Source: CAD feature listing. Evaluate the final solid. Frame: model axes, mm. Face numbers are marked on the shaded views. A direction names the side the tool comes from. Give positions to 0.01 mm unless a question says otherwise; leave off trailing zeros. Order: outer loops, then holes, each group sorted by start corner. A loop starts at its lowest first (then second) coordinate and runs counter-clockwise, first axis right, second up. Notation, with made-up numbers: M 37.5,-13 L 79.5,-13 A22 ccw 79.5,-1 Z; hole C -12.75,-14.5 d1. An arc over 180 degrees is marked long. Use CSV: the item, a comma, the result in double quotes. Start each with the question number.
1. Reachability of the marked faces 5, 6, 7 and 8 from +Z, -Z, +X, -X, +Y, -Y: full face, straight path, thin tool, end or side. Return the list, or none.
2. Section query D-D, the plane z = 5. Return the cut outline in (x, y), plus the area to 3 significant figures.
3. Pin query (flat end, axial travel): P1, Ø12, axis at x = -2.5, y = 20.5, coming from the -Z side; P2, Ø1.5, axis at x = -3.5, z = 15.5, coming from the +Y side; P3, Ø6, axis at y = 12.5, z = 8, coming from the +X side; P4, Ø6.5, axis at y = 9.25, z = 10, coming from the +X side. Return the tip coordinate at first contact, or that it passes through.
4. Section query B-B, the plane y = 42. Return the cut outline in (x, z).
5. Mould query, pull axis Y, two halves, no side actions, for the marked faces 1, 2, 3 and 4. Classes: released by +Y, released by -Y, zero draft, split by the parting line, or undercut.
6. Section query A-A, the plane y = 37. Return the cut outline in (x, z), plus the area to 3 significant figures.
7. Line query: line 1 along X through (y, z) = (43, 14.5); line 2 along Y through (x, z) = (11.5, 16); line 3 along Y through (x, z) = (-15, 16.5). Output: solid intervals per line, ascending. Write a range as [from, to].
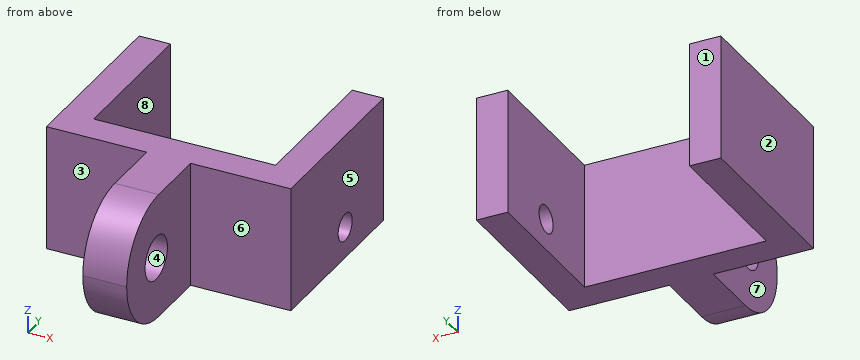
from build123d import *

# Parameters (mm, degrees)
F1_DEPTH = 20
F2_R     = 9.99999
F4_D     = 7
F5_D     = 4.4
F5_DEPTH = 10
F5_TIP   = 1.3218933619


# Not quite as in the source:
# - a fillet or chamfer is up to 0.001 mm smaller than in the source, because OpenCascade refuses the exact size


with BuildPart() as f1:
    # F0 (on Top) → F1 (new body)
    with BuildSketch(Plane.XY):
        Polygon((-18, 49), (-23, 49), (-23, 20), (-7, 20), (-7, 0), (0, 0), (0, 20), (16, 20), (16, 49), (11, 49), (11, 25), (-18, 25), align=None)
    extrude(amount=F1_DEPTH)

    # F2 (radius 10 in the source; OpenCascade refuses exactly that, so slightly less here)
    f2_edges = [f1.edges().sort_by_distance(p)[0] for p in [
        (-3.5, 0, 20),
        (-3.5, 0, 0),
    ]]
    fillet(f2_edges, radius=F2_R)

    # F4 (through all)
    with Locations(Plane.YZ.offset(16)):
        with Locations((9.25, 10)):
            Hole(F4_D / 2)

    # F5
    with Locations(Plane.YZ.offset(16)):
        with Locations((37, 5)):
            Hole(F5_D / 2, depth=F5_DEPTH)
            with Locations((0, 0, -(F5_DEPTH + F5_TIP / 2))):  # 118° drill point
                Cone(0, F5_D / 2, F5_TIP, mode=Mode.SUBTRACT)


solid = f1.part
Result set:
1,face 5,"+Z, -Z, +X, +Y, -Y"
1,face 6,"+Z, -Z, +X, -Y"
1,face 7,"+Z, -Z, -X, -Y"
1,face 8,"+Z, -Z, +Y"
2,outline,"M -23,20 L -7,20 L -7,1.34 L 0,1.34 L 0,20 L 16,20 L 16,34.8 L 11,34.8 L 11,25 L -18,25 L -18,49 L -23,49 Z; M 11,39.2 L 16,39.2 L 16,49 L 11,49 Z"
2,area,"544 mm2"
3,P1,"z = 0"
3,P2,"y = 25"
3,P3,"x = 0"
3,P4,"through"
4,outline,"M -23,0 L -18,0 L -18,20 L -23,20 Z; M 11,0 L 16,0 L 16,20 L 11,20 Z"
5,face 1,"released by +Y"
5,face 2,"zero draft"
5,face 3,"released by -Y"
5,face 4,"undercut"
6,outline,"M -23,0 L -18,0 L -18,20 L -23,20 Z; M 11,0 L 16,0 L 16,2.8 L 11,2.8 Z; M 11,7.2 L 16,7.2 L 16,20 L 11,20 Z"
6,area,"178 mm2"
7,line 1,"[-23, -18], [11, 16]"
7,line 2,"[20, 49]"
7,line 3,"[20, 25]"
